Autodesk Inventor part; units mm, degrees
ref_plane "YZ Plane" through (0, 0, 0) normal (1, 0, 0) x (0, 1, 0)
ref_plane "XZ Plane" through (0, 0, 0) normal (0, 1, 0) x (-1, 0, 0)
ref_plane "XY Plane" through (0, 0, 0) normal (0, 0, 1) x (1, 0, 0)
sketch "Sketch1" plane through (0, 0, 0) normal (0, 0, 1) x (1, 0, 0)
  line L0 (-180, 180) -> (180, 180)
  line L1 (180, 180) -> (180, -180)
  line L2 (180, -180) -> (-180, -180)
  line L3 (-180, -180) -> (-180, 180)
  point P0 (0, 0)
  dimension "d0" = 360
  dimension "d1" = 360
  dimension "d2" = 180
  dimension "d3" = 180
extrude "Extrusion1" add sketch "Sketch1" along normal blind 8
chamfer "Chamfer1" distance 8 angle 45 4 edges at (-180, 0, 8) (0, -180, 8) (180, 0, 8) (0, 180, 8)
sketch "Sketch3" plane through (0, 0, 8) normal (0, 0, 1) x (1, 0, 0)
  line L0 (-172, -172) -> (-172, 172) construction
  line L1 (-172, 142) -> (172, 142) construction
  line L2 (-172, 172) -> (172, 172) construction
  line L3 (-142, 172) -> (-142, -172) construction
  line L4 (172, -172) -> (-172, -172) construction
  line L5 (-172, -142) -> (172, -142) construction
  line L6 (172, 172) -> (172, -172) construction
  line L7 (142, 172) -> (142, -172) construction
  line L8 (-142, 142) -> (-132, 142)
  line L9 (-132, 142) -> (-132, -142)
  line L10 (-132, -142) -> (-142, -142)
  line L11 (-142, -142) -> (-142, 142)
  point P0 (0, 0)
  dimension "d12" = 30
  dimension "d13" = 30
  dimension "d14" = 30
  dimension "d15" = 30
  dimension "d16" = 10
extrude "Extrusion2" cut sketch "Sketch3" against normal blind 5
pattern_linear "Rectangular Pattern1" count 22 spacing 13 along (1, 0, 0) of "Extrusion2"
equation "\"d0\" = edge_length"
equation "\"d1\" = edge_length"
equation "\"d4\" = wall_width"
equation "\"d6\" = wall_width"
equation "\"d12\" = d13"
equation "\"d14\" = d13"
equation "\"d15\" = d13"
properties part number "Element"
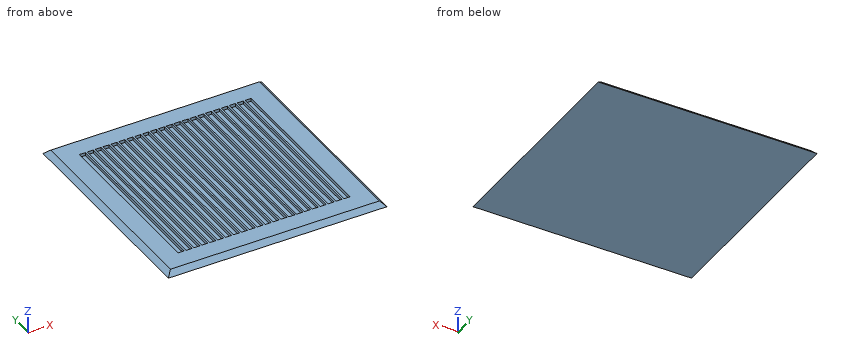
Input: part model. Units: mm. Frame: model coordinates. Round coordinates to 2 decimals unless told otherwise and drop trailing zeros. One line per item, written item: value. Start each with the question number.
(1) Ray query, line 1 (Z direction, x = 9, y = 63); line 2 (Y direction, x = -85, z = 5.25); line 3 (Y direction, x = -96, z = 5.5). Return the intervals inside material, ascending. Write a range as [from, to].
(2) Section A-A, the plane z = 4.5. Count the separate pieces of the cut face and the enclosed holes in it, plus the area to 3 significant figures.
(3) Contact query for flat-ended pins moving along their axis: P1, Ø11, axis at x = 42.5, y = -30.5, coming from the +Z side; P2, Ø2.5, axis at y = -53.5, z = 6.5, coming from the -X side; P3, Ø1.5, axis at x = 6.5, z = 6, coming from the +Y side; P4, Ø1.5, axis at y = 59, z = 5.5, coming from the +X side. Output: stop coordinate, or through.
Results below:
1. line 1: [0, 3]
1. line 2: [-174.75, -142], [142, 174.75]
1. line 3: [-174.5, -142], [142, 174.5]
2. separate pieces: 1
2. enclosed holes: 22
2. area: 60,700 mm^2
3. P1: z = 8
3. P2: x = -174.75
3. P3: y = 174.75
3. P4: x = 175.25
